```python
from build123d import *

# Parameters (mm, degrees)
ESQUISSE1_W                               = 15
ESQUISSE1_H                               = 10
BOSS_EXTRU_1_DEPTH                        = 128
ESQUISSE2_R                               = 3
ENL_V_MAT_EXTRU_1_DEPTH                   = 129.316990301
ENL_V_MAT_EXTRU_2_DEPTH                   = 129.608903269
CHANFREIN1_SIZE                           = 3
TROU_POUR_TARAUDAGE_POUR_TROU_TARAUD_M2_D = 1.6
R_P_TITION_LIN_AIRE1_COUNT                = 3
R_P_TITION_LIN_AIRE1_PITCH                = 61
R_P_TITION_LIN_AIRE1_COUNT_DIR2           = 2
R_P_TITION_LIN_AIRE1_PITCH_DIR2           = 11


with BuildPart() as part:
    # Esquisse1 → Boss.-Extru.1 (new body)
    with BuildSketch(Plane.XY):
        Rectangle(ESQUISSE1_W, ESQUISSE1_H)
    extrude(amount=BOSS_EXTRU_1_DEPTH)

    # Esquisse2 → Enlèv. mat.-Extru.1 (cut, through all)
    with BuildSketch(Plane.XY.offset(128)):
        Circle(ESQUISSE2_R)
    extrude(amount=-ENL_V_MAT_EXTRU_1_DEPTH, mode=Mode.SUBTRACT)

    # Esquisse3 → Enlèv. mat.-Extru.2 (cut, through all)
    with BuildSketch(Plane(origin=(0, 5, 0), x_dir=(1, 0, 0), z_dir=(0, 1, 0))):
        with BuildLine():
            Line((1.55, -16.5), (1.55, -46.5))
            ThreePointArc((1.55, -46.5), (0, -48.05), (-1.55, -46.5))
            Line((-1.55, -46.5), (-1.55, -16.5))
            ThreePointArc((-1.55, -16.5), (0, -14.95), (1.55, -16.5))
        make_face()
    extrude(amount=-ENL_V_MAT_EXTRU_2_DEPTH, mode=Mode.SUBTRACT)

    # Chanfrein1
    chanfrein1_edges = [part.edges().sort_by_distance(p)[0] for p in [
        (-7.5, 5, 64),
        (7.5, 5, 64),
    ]]
    chamfer(chanfrein1_edges, length=CHANFREIN1_SIZE)

    # Trou pour taraudage pour trou taraudé M21 (through all)
    with Locations(Plane(origin=(0, -5, 0), x_dir=(-1, 0, 0), z_dir=(0, -1, 0))):
        with Locations((5.5, -125)):
            trou_pour_taraudage_pour_trou_taraud_m2 = Hole(TROU_POUR_TARAUDAGE_POUR_TROU_TARAUD_M2_D / 2)

    # Répétition linéaire1: Trou pour taraudage pour trou taraud_ M2 3 × 2
    with Locations(*[(j * R_P_TITION_LIN_AIRE1_PITCH_DIR2, 0, -i * R_P_TITION_LIN_AIRE1_PITCH) for i in range(R_P_TITION_LIN_AIRE1_COUNT) for j in range(R_P_TITION_LIN_AIRE1_COUNT_DIR2) if (i, j) != (0, 0)]):
        add(trou_pour_taraudage_pour_trou_taraud_m2, mode=Mode.SUBTRACT)


solid = part.part
```
Work out the finished part from the listing and answer in its coordinate system (mm). A direction names the side the tool comes from. Give positions to 0.01 mm unless a question says otherwise; leave off trailing zeros. Loops run counter-clockwise (first coordinate to the right, second up) from the corner with the lowest first, then second, coordinate; pieces in that order, holes last. Notation, with made-up numbers: (76, 63.25) -> (90, 63.25) arc R38 cw to (90, 101.25) -> close; hole circle Ø5 at (-26.75, -37). An arc over 180 degrees is marked (long way). Put each result on its own line as item: value. Start each with the question number.
Item 1: The mould has two halves that part along X. Classify faces 1 (the face through (-7.5, -2, 63)), 2 (the face through (0, -5, 63)), 3 (the face through (6, 3.5, 63.1)), 4 (the face through (1.55, -4, 31)): released by +X, released by -X, zero draft, split by the parting line, or undercut.
Item 2: Each of these flat-tipped pins is pushed along its axis until it touches: P1, Ø1.2, axis at y = 4, z = 30.5, coming from the -X side; P2, Ø1.8, axis at x = -5.5, z = 125, coming from the +Y side; P3, Ø1.9, axis at y = 3.5, z = 28, coming from the +X side. Where does it stop, or does it pass through?
Item 3: The part is cut by section A-A (x = 0). Give the vertices of the cut face in (y, z), then the cut area to 3 significant figures.
Item 4: The part is cut by section B-B (z = 106). Give the vertices of the cut face in (x, y).
Item 5: Find the intervals of material crossed by L1, parallel to Z at x = 5.5, y = -2.25; L2, parallel to Y at x = 0, z = 48.5; L3, parallel to X at y = 1.75, z = 3, in increasing order. Write a range as [from, to].
Item 6: Which of the six approach directions +Z, -Z, +X, -X, +Y, -Y give full straight-line access (tool end or side, diameter ignored) to faces 5 (the face through (-6, 3.5, 63.1)), 6 (the face through (-1.55, 4, 32))?
Answers below:
1. face 1: released by -X
1. face 2: zero draft
1. face 3: released by +X
1. face 4: undercut
2. P1: x = -6.1
2. P2: y = 4.9
2. P3: x = 6.95
3. outline: (-5, 0) -> (-3, 0) -> (-3, 14.95) -> (-5, 14.95) -> close; (-5, 48.05) -> (-3, 48.05) -> (-3, 128) -> (-5, 128) -> close; (3, 0) -> (5, 0) -> (5, 14.95) -> (3, 14.95) -> close; (3, 48.05) -> (5, 48.05) -> (5, 128) -> (3, 128) -> close
3. area: 380 mm2
4. outline: (-7.5, -5) -> (7.5, -5) -> (7.5, 2) -> (4.5, 5) -> (-4.5, 5) -> (-7.5, 2) -> close; hole circle Ø6 at (0, 0)
5. L1: [0, 2.2], [3.8, 63.2], [64.8, 124.2], [125.8, 128]
5. L2: [-5, -3], [3, 5]
5. L3: [-7.5, -6.3], [-4.7, -2.44], [2.44, 4.7], [6.3, 7.5]
6. face 5: +Z, -Z, -X, +Y
6. face 6: +Y, -Y
